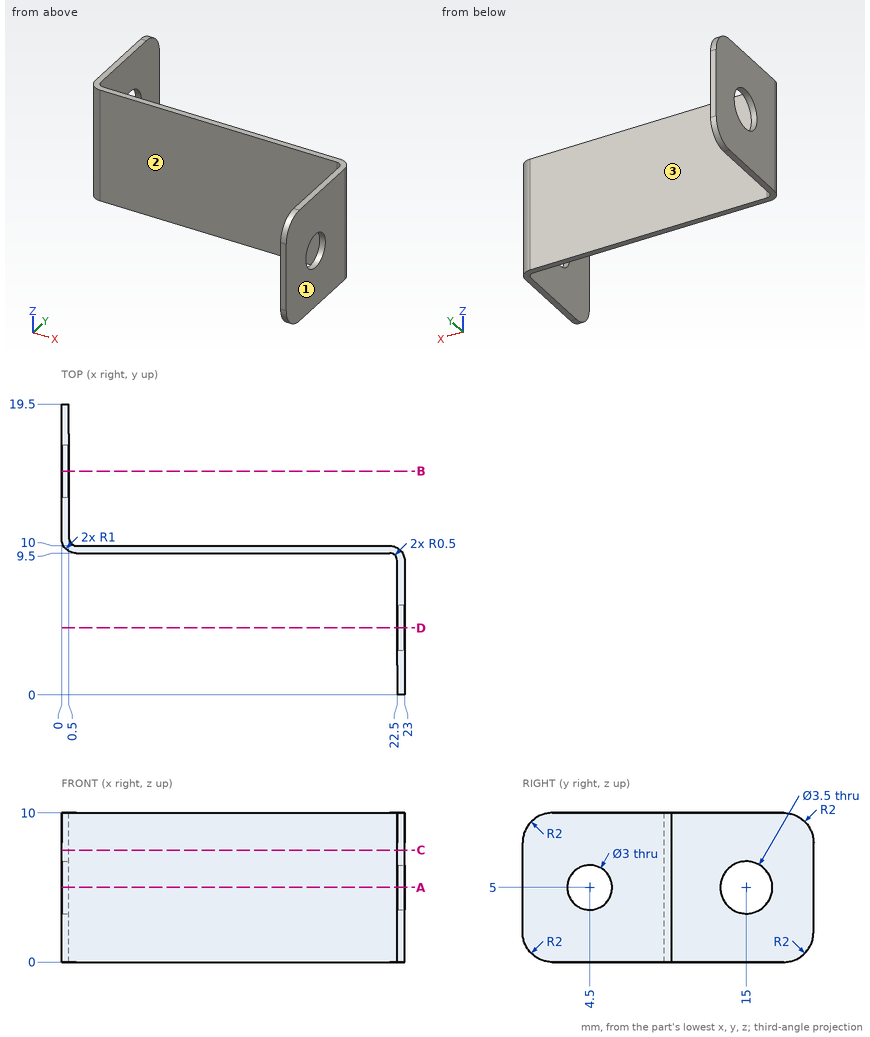
Drawing for the job (mm, zero at the part's lowest x, y, z). A direction names the side the tool comes from. Give positions to 0.01 mm unless a question says otherwise; leave off trailing zeros. Write each loop counter-clockwise with the first axis right and the second up, starting at its lowest first coordinate (ties: lowest second). Pieces come first, ordered by that corner, then holes. Notation, with made-up numbers: M -0.5,2 L 44.5,2 A6 cw 44.5,10 Z; hole C 65,16.5 d7. An arc over 180 degrees is marked long. Return JSON: item names as keys, results as strings. Group by question number.
(1) Band-saw the part on D-D (y = 4.5). Give the cut face in (x, z).
(2) 3-axis set-ups, long thin cutter, end or side, ignore diameter. For the marked faces 1, 2 and 3: which of +Z, -Z, +X, -X, +Y, -Y reach the whole face in a straight line?
(3) Band-saw the part on C-C (z = 7.5). Give the cut face in (x, y), and give its area (3 significant figures).
(4) Drill centre lines: L1, parallel to Z at x = 0.1, y = 15; L2, parallel to Z at x = 22.65, y = 4.5; L3, parallel to Y at x = 20.25, z = 3.25. Where is each one in solid material? Low to high. Write a range as [from, to].
(5) Flat gauge pins, fed straight in: pin 1 Ø4 at (x, z) = (14, 8.5) entering from +Y; pin 2 Ø2.5 at (y, z) = (4.5, 5) entering from -X; pin 3 Ø2.5 at (y, z) = (14, 4.5) entering from +X. Where does each tip first touch, or does it go through?
(6) Band-saw the part on A-A (z = 5). Give the cut face in (x, y).
(7) Band-saw the part on B-B (y = 15). Give the cut face in (x, z), and give its area (3 significant figures).
Entries:
{
 "1": {"outline": "M 22.5,0 L 23,0 L 23,3.5 L 22.5,3.5 Z; M 22.5,6.5 L 23,6.5 L 23,10 L 22.5,10 Z"},
 "2": {"face 1": "+Z, -Z, +X, +Y, -Y", "face 2": "+Z, -Z, -X, -Y", "face 3": "+Z, -Z, +X, +Y"},
 "3": {"outline": "M 0,10.5 A1 ccw 1,9.5 L 22,9.5 A0.5 cw 22.5,9 L 22.5,0 L 23,0 L 23,9 A1 ccw 22,10 L 1,10 A0.5 cw 0.5,10.5 L 0.5,19.5 L 0,19.5 Z", "area": "20.7 mm^2"},
 "4": {"L1": "z = [0, 3.25], [6.75, 10]", "L2": "z = [0, 3.5], [6.5, 10]", "L3": "y = [9.5, 10]"},
 "5": {"pin 1": "stops at y = 10", "pin 2": "passes through", "pin 3": "stops at x = 0.5"},
 "6": {"outline": "M 0,10.5 A1 ccw 1,9.5 L 22,9.5 A0.5 cw 22.5,9 L 22.5,6 L 23,6 L 23,9 A1 ccw 22,10 L 1,10 A0.5 cw 0.5,10.5 L 0.5,13.25 L 0,13.25 Z; M 0,16.75 L 0.5,16.75 L 0.5,19.5 L 0,19.5 Z; M 22.5,0 L 23,0 L 23,3 L 22.5,3 Z"},
 "7": {"outline": "M 0,0 L 0.5,0 L 0.5,3.25 L 0,3.25 Z; M 0,6.75 L 0.5,6.75 L 0.5,10 L 0,10 Z", "area": "3.25 mm^2"}
}
